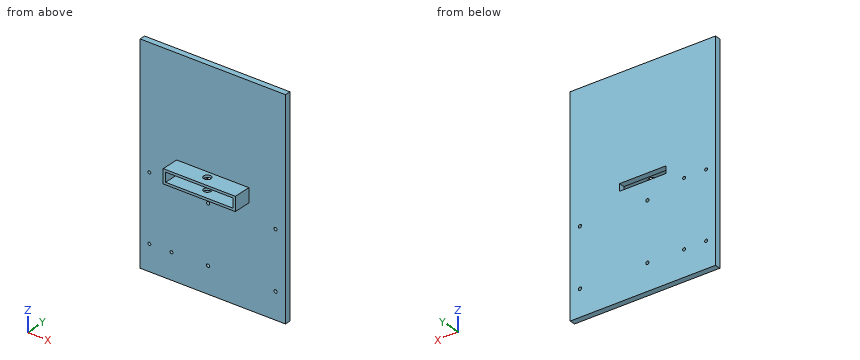
from build123d import *

# Parameters (mm, degrees)
ESQUISSE1_W                  = 62
ESQUISSE1_H                  = 12
ESQUISSE1_W_2                = 58
ESQUISSE1_H_2                = 8
BOSS_EXTRU_1_DEPTH           = 15
ESQUISSE2_R                  = 3.175
ENL_V_MAT_EXTRU_1_DEPTH      = 37.469165058
ESQUISSE3_W                  = 125
ESQUISSE3_H                  = 180
BOSS_EXTRU_2_DEPTH           = 5
ENL_V_MAT_EXTRU_3_REACH      = 112.595
ESQUISSE6_W                  = 40
ESQUISSE6_H                  = 6
ENL_V_MAT_EXTRU_4_DEPTH      = 112.38334705
ENL_V_MAT_EXTRU_4_DEPTH_BACK = 112.38334705
ESQUISSE8_R                  = 1.375
ENL_V_MAT_EXTRU_5_DEPTH      = 112.38334705
ENL_V_MAT_EXTRU_5_DEPTH_BACK = 112.38334705
ESQUISSE9_R                  = 1.25


with BuildPart() as part:
    # Esquisse1 → Boss.-Extru.1 (new body)
    with BuildSketch(Plane(origin=(0, 0, 0), x_dir=(1, 0, 0), z_dir=(0, 1, 0))):
        Rectangle(ESQUISSE1_W, ESQUISSE1_H)
        Rectangle(ESQUISSE1_W_2, ESQUISSE1_H_2, mode=Mode.SUBTRACT)
    extrude(amount=BOSS_EXTRU_1_DEPTH)

    # Esquisse2 → Enlèv. mat.-Extru.1 (cut, through all)
    with BuildSketch(Plane.XY.offset(6)):
        with Locations((0, 9)):
            Circle(ESQUISSE2_R)
    extrude(amount=-ENL_V_MAT_EXTRU_1_DEPTH, mode=Mode.SUBTRACT)

    # Esquisse3 → Boss.-Extru.2 (add)
    with BuildSketch(Plane(origin=(0, 15, 0), x_dir=(1, 0, 0), z_dir=(0, 1, 0))):
        Rectangle(ESQUISSE3_W, ESQUISSE3_H)
    extrude(amount=BOSS_EXTRU_2_DEPTH)

    # Esquisse6 → Enlèv. mat.-Extru.3 (cut, up to next)
    with BuildSketch(Plane(origin=(0, 15, 0), x_dir=(-1, 0, 0), z_dir=(0, -1, 0)), mode=Mode.PRIVATE) as enl_v_mat_extru_3_sk1:
        Rectangle(ESQUISSE6_W, ESQUISSE6_H)
    enl_v_mat_extru_3_tool1 = extrude(enl_v_mat_extru_3_sk1.sketch, amount=-ENL_V_MAT_EXTRU_3_REACH, mode=Mode.PRIVATE) & part.part
    add(enl_v_mat_extru_3_tool1.solids().sort_by_distance((0, 15, 0))[0], mode=Mode.SUBTRACT)

    # Esquisse8 → Enlèv. mat.-Extru.4 (cut, two sides: drawn at the far end of the back side and taken through both)
    with BuildSketch(Plane(origin=(0, 20, 0), x_dir=(1, 0, 0), z_dir=(0, 1, 0)).offset(-ENL_V_MAT_EXTRU_4_DEPTH_BACK)):
        with Locations(Location((54, 67.5, 0), (0, 0, 270))):
            Circle(ESQUISSE8_R)
        with Locations(Location((54, 18.5, 0), (0, 0, 270))):
            Circle(ESQUISSE8_R)
        with Locations(Location((-4, 67.5, 0), (0, 0, 270))):
            Circle(ESQUISSE8_R)
        with Locations(Location((-4, 18.5, 0), (0, 0, 270))):
            Circle(ESQUISSE8_R)
    extrude(amount=ENL_V_MAT_EXTRU_4_DEPTH + ENL_V_MAT_EXTRU_4_DEPTH_BACK, mode=Mode.SUBTRACT)

    # Esquisse9 → Enlèv. mat.-Extru.5 (cut, two sides: drawn at the far end of the back side and taken through both)
    with BuildSketch(Plane(origin=(0, 20, 0), x_dir=(1, 0, 0), z_dir=(0, 1, 0)).offset(-ENL_V_MAT_EXTRU_5_DEPTH_BACK)):
        with Locations(Location((-35.5, 68, 0), (0, 0, 270))):
            Circle(ESQUISSE9_R)
        with Locations(Location((-54.5, 68, 0), (0, 0, 270))):
            Circle(ESQUISSE9_R)
        with Locations(Location((-35.5, 12, 0), (0, 0, 270))):
            Circle(ESQUISSE9_R)
        with Locations(Location((-54.5, 12, 0), (0, 0, 270))):
            Circle(ESQUISSE9_R)
    extrude(amount=ENL_V_MAT_EXTRU_5_DEPTH + ENL_V_MAT_EXTRU_5_DEPTH_BACK, mode=Mode.SUBTRACT)


solid = part.part
The model under review builds one solid part; all positions refer to its coordinate system, in mm. Coordinates: 2 decimals unless noted, no trailing zeros. Write each loop counter-clockwise with the first axis right and the second up, starting at its lowest first coordinate (ties: lowest second). Pieces come first, ordered by that corner, then holes. Notation, with made-up numbers: (47, 3.25) -> (86, 3.25) arc R17 cw to (86, 13.25) -> close; hole circle Ø1 at (8, 36.25). An arc over 180 degrees is marked (long way). Answer in a Markdown table with one row per item.
1. We need section D-D, the plane x = 49.5. State the section outline as (y, z) points, and give its area (3 significant figures).
Answers below:
| item | result |
|---|---|
| outline | (15, -90) -> (20, -90) -> (20, 90) -> (15, 90) -> close |
| area | 900 mm^2 |
2. We need section C-C, the plane z = 40. State the section outline as (x, y) points.
Answers below:
| item | result |
|---|---|
| outline | (-62.5, 15) -> (62.5, 15) -> (62.5, 20) -> (-62.5, 20) -> close |
3. We need section A-A, the plane y = 9. State the section outline as (x, z) points (3 decimals), and give its area (3 significant figures).
Answers below:
| item | result |
|---|---|
| outline | (-31, -6) -> (-3.175, -6) -> (-3.175, -4) -> (-29, -4) -> (-29, 4) -> (-3.175, 4) -> (-3.175, 6) -> (-31, 6) -> close; (3.175, -6) -> (31, -6) -> (31, 6) -> (3.175, 6) -> (3.175, 4) -> (29, 4) -> (29, -4) -> (3.175, -4) -> close |
| area | 255 mm^2 |
4. We need section B-B, the plane x = -14.5. State the section outline as (y, z) points.
Answers below:
| item | result |
|---|---|
| outline | (0, -6) -> (15, -6) -> (15, -90) -> (20, -90) -> (20, -3) -> (15, -3) -> (15, -4) -> (0, -4) -> close; (0, 4) -> (15, 4) -> (15, 3) -> (20, 3) -> (20, 90) -> (15, 90) -> (15, 6) -> (0, 6) -> close |
5. Wall thickness on probe 1 along X at (y, z) = (18.4, -18.5) (3 decimals); probe 2 along Z at (x, y) = (-35.5, 17.95); probe 3 along Z at (x, y) = (-4, 17.6) (3 decimals): over which ranges is each line inside the solid? List them lowest first. Write a range as [from, to].
Answers below:
| item | result |
|---|---|
| probe 1 | x = [-62.5, -5.375], [-2.625, 52.625], [55.375, 62.5] |
| probe 2 | z = [-90, -69.25], [-66.75, -13.25], [-10.75, 90] |
| probe 3 | z = [-90, -68.875], [-66.125, -19.875], [-17.125, -3], [3, 90] |
6. Clearance check with flat-ended pins moving along their axes: pin 1 Ø6 at (x, y) = (-16.5, 11) entering from +Z; pin 2 Ø5 at (y, z) = (10.5, -19) entering from +X; pin 3 Ø3 at (x, z) = (54, -67.5) entering from -Y; pin 4 Ø1.5 at (x, y) = (22.5, 13.5) entering from -Z. State where each tip first meets the part, or that it passes through.
Answers below:
| item | result |
|---|---|
| pin 1 | stops at z = 6 |
| pin 2 | passes through |
| pin 3 | stops at y = 15 |
| pin 4 | stops at z = -6 |
